Autodesk Inventor part; units mm, degrees
ref_plane "YZ Plane" through (0, 0, 0) normal (1, 0, 0) x (0, 1, 0)
ref_plane "XZ Plane" through (0, 0, 0) normal (0, 1, 0) x (-1, 0, 0)
ref_plane "XY Plane" through (0, 0, 0) normal (0, 0, 1) x (1, 0, 0)
sketch "スケッチ2" plane through (0, 0, 0) normal (1, 0, 0) x (0, 1, 0)
  line L0 (25, 10) -> (-25, 10)
  line L1 (-25, 10) -> (-25, -10)
  line L2 (-25, -10) -> (25, -10)
  line L3 (25, -10) -> (25, 10)
  line L4 (25, 10) -> (-25, -10) construction
  line L5 (-25, 10) -> (25, -10) construction
  point P0 (0, 0)
  dimension "d4" = 50
  dimension "d5" = 20
extrude "押し出し2" add sketch "スケッチ2" along normal mid plane 500
sketch "スケッチ3" plane through (-250, -25, 10) normal (0, 0, 1) x (1, 0, 0)
  circle A0 centre (250, 25) radius 5
  dimension "d8" = 10
extrude "押し出し3" add sketch "スケッチ3" along normal blind 2
fillet "フィレット1" radius 2 2 edges at (250, 0, -10) (-250, 0, -10)
sketch "スケッチ4" plane through (250, 0, 0) normal (1, 0, 0) x (0, 0, -1)
  line L0 (-6, 21) -> (6, 21)
  line L1 (6, 21) -> (6, -21)
  line L2 (6, -21) -> (-6, -21)
  line L3 (-6, -21) -> (-6, 21)
  line L4 (-6, 21) -> (6, -21) construction
  line L5 (6, 21) -> (-6, -21) construction
  point P0 (0, 0)
  dimension "d12" = 12
  dimension "d13" = 42
extrude "押し出し4" cut sketch "スケッチ4" against normal through all
properties part number "hashi1shado"
Here's how the part is built. I have some questions about the finished solid (model axes, mm). A direction names the side the tool comes from. Give positions to 0.01 mm unless a question says otherwise; leave off trailing zeros. Write each loop counter-clockwise with the first axis right and the second up, starting at its lowest first coordinate (ties: lowest second). Pieces come first, ordered by that corner, then holes. Notation, with made-up numbers: M -10,71 L 7,71 A7 cw 7,83 Z; hole C 49.25,47.5 d4. An arc over 180 degrees is marked long. Put each result on its own line as item: value. Start each with the question number.
Item 1: I need wall thicknesses on L1, parallel to Z at x = 228.5, y = -20.5; L2, parallel to Y at x = -89, z = -5.5; L3, parallel to X at y = 17, z = -8.5. Which ranges of each line are inside material? Lowest first, please. Write a range as from..to.
Item 2: Will this pin go through, and if not, where does the flat tip stop? pin 1 (3 mm diameter, centred on x = -162.5, y = 0, fed in from +Z).
Item 3: If we section it at C-C, the plane x = 0: Write out the boundary of the cut face in (y, z).
Item 4: If we section it at D-D, the plane x = -81: Write out the boundary of the cut face in (y, z), then the cut area to 3 significant figures.
Item 5: If we section it at B-B, the plane y = 0: Write out the boundary of the cut face in (x, z), then the cut area to 3 significant figures.
Item 6: If we section it at A-A, the plane z = 1: Write out the boundary of the cut face in (x, y), then the cut area to 3 significant figures.
Item 7: Thinking about a two-plate mould opening in Z: for faces 3 (the flat face through (-4, 6, 10)), 4 (the cylindrical face through (-1.08, 4.88, 10.99)), 5 (the flat face through (4, 21, 0)), which applies, +Z half, -Z half, draft (parallel to the pull), parting line (faces both ways), or undercut?
Item 8: On a 3-axis mill with a long thin cutter (end or side, diameter ignored), from which of +Z, -Z, +X, -X, +Y, -Y can I reach the whole of each face in a straight line? I mean faces 1 (the flat face through (-4, 25, 0)), 2 (the flat face through (4, 0, -6)). Say none if no direction works.
Values:
1. L1: -10..-6, 6..10
1. L2: -25..-21, 21..25
1. L3: -249.94..249.94
2. pin 1: z = 10
3. outline: M -25,-10 L 25,-10 L 25,10 L 5,10 L 5,12 L -5,12 L -5,10 L -25,10 Z; hole M -21,-6 L 21,-6 L 21,6 L -21,6 Z
4. outline: M -25,-10 L 25,-10 L 25,10 L -25,10 Z; hole M -21,-6 L 21,-6 L 21,6 L -21,6 Z
4. area: 496 mm²
5. outline: M -250,-8 A2 ccw -248,-10 L 248,-10 A2 ccw 250,-8 L 250,-6 L -250,-6 Z; M -250,6 L 250,6 L 250,10 L 5,10 L 5,12 L -5,12 L -5,10 L -250,10 Z
5. area: 4,020 mm²
6. outline: M -250,-25 L 250,-25 L 250,-21 L -250,-21 Z; M -250,21 L 250,21 L 250,25 L -250,25 Z
6. area: 4,000 mm²
7. face 3: +Z half
7. face 4: draft
7. face 5: undercut
8. face 1: +Z, -Z, +X, -X, +Y
8. face 2: +X, -X
